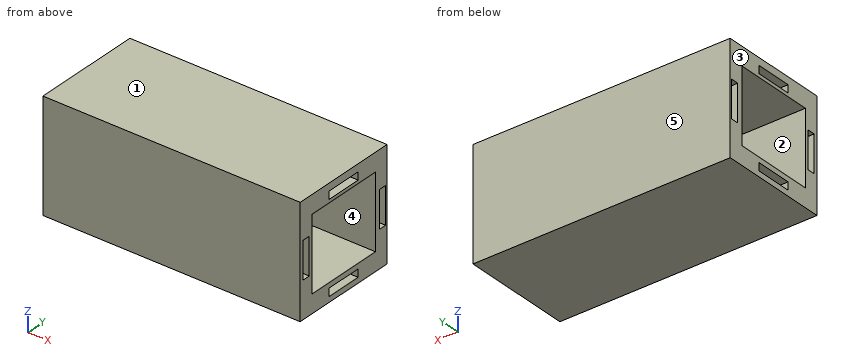
Autodesk Fusion 360 part; units mm, degrees
sketch "Sketch1" plane through (0, 0, 0) normal (1, 0, 0) x (0, 1, 0)
  line L0 (0, 0) -> (30, 0)
  line L1 (30, 0) -> (30, 30)
  line L2 (30, 30) -> (0, 30)
  line L3 (0, 30) -> (0, 0)
  line L4 (1, 20) -> (3.1, 20)
  line L5 (3.1, 20) -> (3.1, 10)
  line L6 (3.1, 10) -> (1, 10)
  line L7 (1, 10) -> (1, 20)
  line L8 (10, 28) -> (20, 28)
  line L9 (20, 28) -> (20, 25.9)
  line L10 (20, 25.9) -> (10, 25.9)
  line L11 (10, 25.9) -> (10, 28)
  line L12 (29.5, 19.9621) -> (27.4, 19.9621)
  line L13 (27.4, 19.9621) -> (27.4, 9.9621)
  line L14 (27.4, 9.9621) -> (29.5, 9.9621)
  line L15 (29.5, 9.9621) -> (29.5, 19.9621)
  line L16 (10, 1.5) -> (20, 1.5)
  line L17 (20, 1.5) -> (20, 3.6)
  line L18 (20, 3.6) -> (10, 3.6)
  line L19 (10, 3.6) -> (10, 1.5)
  line L20 (4, 25) -> (26, 25)
  line L21 (26, 25) -> (26, 5)
  line L22 (26, 5) -> (4, 5)
  line L23 (4, 5) -> (4, 25)
  dimension "d1" = 30
  dimension "d2" = 30
  dimension "d3" = 2.1
  dimension "d4" = 10
  dimension "d5" = 10
  dimension "d6" = 2.1
  dimension "d7" = 2.1
  dimension "d8" = 10
  dimension "d9" = 0.5
  dimension "d10" = 10
  dimension "d11" = 2.1
  dimension "d12" = 1.5
extrude "Extrude1" add sketch "Sketch1" along normal blind 70
Can you work these out from the model? Positions are in its coordinate system, mm. Face numbers are marked on the shaded views. A direction names the side the tool comes from. Give positions to 0.01 mm unless a question says otherwise; leave off trailing zeros. Loops run counter-clockwise (first coordinate to the right, second up) from the corner with the lowest first, then second, coordinate; pieces in that order, holes last. Notation, with made-up numbers: (-1, 34.25) - (43, 34.25) arc R18 ccw to (43, 63.25) - close; hole circle Ø10 at (30, 77). An arc over 180 degrees is marked (long way). Answer as a JSON object with one key per item and string values.
Q1. If I drill on L1, parallel to Z at x = 38, y = 11.75; L2, parallel to Y at x = 27, z = 18.25; L3, parallel to Z at x = 50, y = 2.25, over which ranges is the centre line in solid material (lowest first)?
Geometry says:
{"L1": "0 to 1.5, 3.6 to 5, 25 to 25.9, 28 to 30", "L2": "0 to 1, 3.1 to 4, 26 to 27.4, 29.5 to 30", "L3": "0 to 10, 20 to 30"}
Q2. Imagine slicing it at D-D on z = 7. Write out the boundary of the cut face in (x, y).
Geometry says:
{"outline": "(0, 0) - (70, 0) - (70, 4) - (0, 4) - close; (0, 26) - (70, 26) - (70, 30) - (0, 30) - close"}
Q3. Will this pin go through, and if not, where does the flat tip stop? P1, Ø2.5, axis at x = 23, z = 2.5, coming from the -Y side.
Geometry says:
{"P1": "y = 0"}
Q4. Imagine slicing it at C-C on y = 17.25. Write out the boundary of the cut face in (x, z), plus the area to 3 significant figures.
Geometry says:
{"outline": "(0, 0) - (70, 0) - (70, 1.5) - (0, 1.5) - close; (0, 3.6) - (70, 3.6) - (70, 5) - (0, 5) - close; (0, 25) - (70, 25) - (70, 25.9) - (0, 25.9) - close; (0, 28) - (70, 28) - (70, 30) - (0, 30) - close", "area": "406 mm²"}
Q5. Which directions (+Z, -Z, +X, -X, +Y, -Y) give clear straight access to the entire face, cutting with the end or side of a thin tool? Please do the marked faces 4 and 5.
Geometry says:
{"face 4": "+X, -X", "face 5": "+Z, -Z, +X, -X, +Y"}
Q6. Imagine slicing it at B-B on z = 14.25. Write out the boundary of the cut face in (x, y).
Geometry says:
{"outline": "(0, 0) - (70, 0) - (70, 1) - (0, 1) - close; (0, 3.1) - (70, 3.1) - (70, 4) - (0, 4) - close; (0, 26) - (70, 26) - (70, 27.4) - (0, 27.4) - close; (0, 29.5) - (70, 29.5) - (70, 30) - (0, 30) - close"}
Q7. If we mould it in two halves opening along Z, with no side actions, what happens to the marked faces 1, 2 and 3? For each: pulls with the +Z half, pulls with the -Z half, needs draft (parallel to the pull), parting line crosses it, or undercut.
Geometry says:
{"face 1": "pulls with the +Z half", "face 2": "undercut", "face 3": "needs draft"}
Q8. Imagine slicing it at A-A on y = 8.5. Write out the boundary of the cut face in (x, z).
Geometry says:
{"outline": "(0, 0) - (70, 0) - (70, 5) - (0, 5) - close; (0, 25) - (70, 25) - (70, 30) - (0, 30) - close"}
